from build123d import *

# Parameters (mm, degrees)
SKETCH2_R           = 1.5
BOSS_EXTRUDE1_DEPTH = 10
SKETCH3_W           = 25
SKETCH3_H           = 40
SKETCH3_W_2         = 40
SKETCH3_H_2         = 25
BOSS_EXTRUDE2_DEPTH = 40
CUT_EXTRUDE1_DEPTH  = 40
CIRPATTERN1_COUNT   = 4


with BuildPart() as part:
    # Sketch2 → Boss-Extrude1 (new body)
    with BuildSketch(Plane(origin=(0, 0, 0), x_dir=(1, 0, 0), z_dir=(0, 1, 0))):
        with BuildLine():
            Line((162.66, -17.328961432), (162.66, 17.328961432))
            ThreePointArc((162.66, 17.328961432), (56.705609793, 56.705609793), (17.328961432, 162.66))
            Line((17.328961432, 162.66), (-17.328961432, 162.66))
            ThreePointArc((-17.328961432, 162.66), (-56.705609793, 56.705609793), (-162.66, 17.328961432))
            Line((-162.66, 17.328961432), (-162.66, -17.328961432))
            ThreePointArc((-162.66, -17.328961432), (-56.705609793, -56.705609793), (-17.328961432, -162.66))
            Line((-17.328961432, -162.66), (17.328961432, -162.66))
            ThreePointArc((17.328961432, -162.66), (56.705609793, -56.705609793), (162.66, -17.328961432))
        make_face()
        with Locations((-12, -157.66)):
            Circle(SKETCH2_R, mode=Mode.SUBTRACT)
        with Locations((-157.66, -12)):
            Circle(SKETCH2_R, mode=Mode.SUBTRACT)
        with Locations((12, -157.66)):
            Circle(SKETCH2_R, mode=Mode.SUBTRACT)
        with Locations((157.66, -12)):
            Circle(SKETCH2_R, mode=Mode.SUBTRACT)
        with Locations((-157.66, 12)):
            Circle(SKETCH2_R, mode=Mode.SUBTRACT)
        with Locations((-12, 157.66)):
            Circle(SKETCH2_R, mode=Mode.SUBTRACT)
        with Locations((157.66, 12)):
            Circle(SKETCH2_R, mode=Mode.SUBTRACT)
        with Locations((12, 157.66)):
            Circle(SKETCH2_R, mode=Mode.SUBTRACT)
    extrude(amount=BOSS_EXTRUDE1_DEPTH)

    # Sketch3 → Boss-Extrude2 (add)
    with BuildSketch(Plane.XZ):
        with Locations((0, 127.465698487)):
            Rectangle(SKETCH3_W, SKETCH3_H)
        with Locations((127.465698487, 0)):
            Rectangle(SKETCH3_W_2, SKETCH3_H_2)
        with Locations((0, -127.465698487)):
            Rectangle(SKETCH3_W, SKETCH3_H)
        with Locations((-127.465698487, 0)):
            Rectangle(SKETCH3_W_2, SKETCH3_H_2)
    extrude(amount=BOSS_EXTRUDE2_DEPTH)

    # Sketch4 → Cut-Extrude1 (cut)
    with BuildSketch(Plane(origin=(0, 0, -12.5), x_dir=(-1, 0, 0), z_dir=(0, 0, -1))):
        Polygon((-131.465698487, -40), (-107.465698487, 0), (-107.465698487, -40), align=None)
    cut_extrude1 = extrude(amount=-CUT_EXTRUDE1_DEPTH, mode=Mode.SUBTRACT)

    # CirPattern1: Cut-Extrude1 ×4 about axis
    cirpattern1_axis = Axis((0, 0, 0), (0, 1, 0))
    for i in range(1, CIRPATTERN1_COUNT):
        add(cut_extrude1.rotate(cirpattern1_axis, i * 360 / CIRPATTERN1_COUNT), mode=Mode.SUBTRACT)


solid = part.part
Here's how the part is built. I have some questions about the finished solid (model axes, mm). A direction names the side the tool comes from. Coordinates: 2 decimals unless noted, no trailing zeros. Loops run counter-clockwise (first coordinate to the right, second up) from the corner with the lowest first, then second, coordinate; pieces in that order, holes last.
1. Imagine slicing it at D-D, the plane y = -16. Please give me the cut outline in (x, z), and give its area (3 significant figures).
2. I need wall thicknesses on L1, parallel to Z at x = -12, y = 5.75; L2, parallel to Z at x = 157, y = 7; L3, parallel to X at y = 3.5, z = -157.66. Which ranges of each line are inside material? Lowest first, please.
3. Imagine slicing it at B-B, the plane z = -5. Please give me the cut outline in (x, y).
4. Imagine slicing it at A-A, the plane y = -35. Please give me the cut outline in (x, z), and give its area (3 significant figures).
5. For P1, Ø20, axis at y = -26.5, z = 6, coming from the +X side; P2, Ø4, axis at x = 157.66, z = -12, coming from the +Y side; P3, Ø7.5, axis at x = 5, y = -13, coming from the +Z side; P4, Ø5, axis at x = 12, z = -157.66, coming from the -Y side, each with a flat end and sliding along its axis, tell me the tip position at first contact or that it passes through.
6. Imagine slicing it at C-C, the plane x = -119. Please give me the cut outline in (y, z).
7. For faces 1 (the flat face through (-0.175, -20.28, -119.634)), 2 (the flat face through (-119.634, -20.28, 0.175)), 3 (the flat face through (132, -15, -12.5)), 4 (the flat face through (-12.5, -15, 132)), which set-ups out of +Z, -Z, +X, -X, +Y, -Y let a thin tool reach every point of the face, with its end or its side?
8. If we mould it in two halves opening along X, with no side actions, what happens to faces 5 (the flat face through (12.5, -15, -132)), 6 (the flat face through (119.634, -20.28, -0.175)), 7 (the flat face through (0, -20, -147.466))? For each: pulls with the +X half, pulls with the -X half, needs draft (parallel to the pull), parting line crosses it, or undercut.
Taken from the geometry:
1. outline: (-147.47, -12.5) - (-117.07, -12.5) - (-117.07, 12.5) - (-147.47, 12.5) - close; (-12.5, -147.47) - (12.5, -147.47) - (12.5, -117.07) - (-12.5, -117.07) - close; (-12.5, 117.07) - (12.5, 117.07) - (12.5, 147.47) - (-12.5, 147.47) - close; (117.07, -12.5) - (147.47, -12.5) - (147.47, 12.5) - (117.07, 12.5) - close
1. area: 3,040 mm2
2. L1: z = -162.66 to -159.16, -156.16 to 156.16, 159.16 to 162.66
2. L2: z = -17.03 to -13.35, -10.65 to 10.65, 13.35 to 17.03
2. L3: x = -17.05 to -13.5, -10.5 to 10.5, 13.5 to 17.05
3. outline: (-162.66, 0) - (-147.47, 0) - (-147.47, -40) - (-131.47, -40) - (-107.47, 0) - (107.47, 0) - (131.47, -40) - (147.47, -40) - (147.47, 0) - (162.66, 0) - (162.66, 10) - (-162.66, 10) - close
4. outline: (-147.47, -12.5) - (-128.47, -12.5) - (-128.47, 12.5) - (-147.47, 12.5) - close; (-12.5, -147.47) - (12.5, -147.47) - (12.5, -128.47) - (-12.5, -128.47) - close; (-12.5, 128.47) - (12.5, 128.47) - (12.5, 147.47) - (-12.5, 147.47) - close; (128.47, -12.5) - (147.47, -12.5) - (147.47, 12.5) - (128.47, 12.5) - close
4. area: 1,900 mm2
5. P1: stops at x = 147.47
5. P2: stops at y = 10
5. P3: stops at z = 147.47
5. P4: stops at y = 0
6. outline: (-19.22, -12.5) - (0, -12.5) - (0, -21.2) - (10, -21.2) - (10, 21.2) - (0, 21.2) - (0, 12.5) - (-19.22, 12.5) - close
7. face 1: +X, -X, -Y
7. face 2: +Z, -Z, -Y
7. face 3: -Z, +X, -X, -Y
7. face 4: +Z, -Z, -X, -Y
8. face 5: pulls with the +X half
8. face 6: undercut
8. face 7: needs draft
